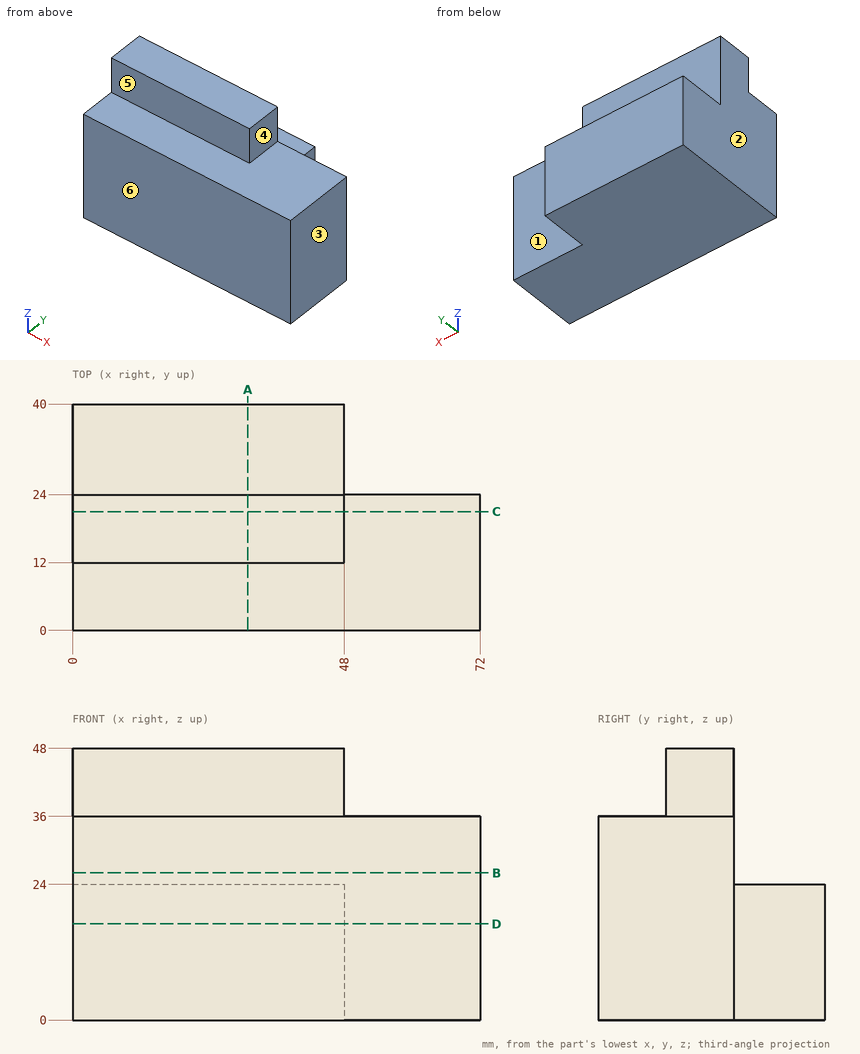
Could you check a few things on this drawing? It's one solid part, dimensions in mm from its lowest x, y, z. A direction names the side the tool comes from. Give positions to 0.01 mm unless a question says otherwise; leave off trailing zeros. Write each loop counter-clockwise with the first axis right and the second up, starting at its lowest first coordinate (ties: lowest second). Pieces come first, ordered by that corner, then holes. Notation, with made-up numbers: (88.25, 36.5) -> (124.25, 36.5) arc R17 ccw to (124.25, 63.5) -> close; hole circle Ø7 at (75.25, 64). An arc over 180 degrees is marked (long way). Write item = value, one per line.
(1) Suppose I cut it at C-C on y = 21. Write out the boundary of the cut face in (x, z), then the cut area to 3 significant figures.
Worked out:
outline = (0, 0) -> (72, 0) -> (72, 36) -> (48, 36) -> (48, 48) -> (0, 48) -> close
area = 3,170 mm^2
(2) Suppose I cut it at A-A on x = 31. Write out the boundary of the cut face in (y, z).
Worked out:
outline = (0, 0) -> (40, 0) -> (40, 24) -> (24, 24) -> (24, 48) -> (12, 48) -> (12, 36) -> (0, 36) -> close
(3) For the marked faces 4, 5 and 6, which set-ups out of +Z, -Z, +X, -X, +Y, -Y let a thin tool reach every point of the face, with its end or its side?
Worked out:
face_4 = +Z, +X, +Y, -Y
face_5 = +Z, +X, -X, -Y
face_6 = +Z, -Z, +X, -X, -Y
(4) Suppose I cut it at B-B on z = 26. Write out the boundary of the cut face in (x, y).
Worked out:
outline = (0, 0) -> (72, 0) -> (72, 24) -> (0, 24) -> close
(5) Thinking about a two-plate mould opening in X: for the marked faces 1, 2 and 3, which applies, released by +X, released by -X, zero draft, split by the parting line, or undercut?
Worked out:
face_1 = zero draft
face_2 = released by -X
face_3 = released by +X
(6) Suppose I cut it at D-D on z = 17. Write out the boundary of the cut face in (x, y), then the cut area to 3 significant figures.
Worked out:
outline = (0, 0) -> (72, 0) -> (72, 24) -> (48, 24) -> (48, 40) -> (0, 40) -> close
area = 2,500 mm^2
(7) I need wall thicknesses on probe 1 along Y at (x, z) = (13, 28); probe 2 along X at (y, z) = (29, 10). Which ranges of each line are inside material? Lowest first, please. Write a range as from..to.
Worked out:
probe_1 = 0..24
probe_2 = 0..48
(8) I'm going to push flat-ended pins straight in: P1, Ø6, axis at x = 24.5, z = 42, coming from the -Y side; P2, Ø8, axis at y = 28.5, z = 9.5, coming from the +X side. Where does each tip first touch, or does it pass through?
Worked out:
P1 = 12
P2 = 48
